Work out the finished part from the listing and answer in its coordinate system (mm). A direction names the side the tool comes from. Give positions to 0.01 mm unless a question says otherwise; leave off trailing zeros. Write each loop counter-clockwise with the first axis right and the second up, starting at its lowest first coordinate (ties: lowest second). Pieces come first, ordered by that corner, then holes. Notation, with made-up numbers: (19.25, 43.5) -> (37.25, 43.5) arc R28 cw to (37.25, 63.5) -> close; hole circle Ø8 at (76, 67.25). An arc over 180 degrees is marked (long way). Use a Markdown table: item, result. Add a question column.
Q1. For a pull along Z with two mould halves and no side action, classify faces 1 (the face through (9.63, 2.69, 22.18)), 2 (the face through (6, 6, 0)), 3 (the face through (6, 6, 35)) as pulls with the +Z half, pulls with the -Z half, needs draft (parallel to the pull), parting line crosses it, or undercut.
Q2. For faces 4 (the face through (9, 2.3, 24.4)), 5 (the face through (1.78, 9.22, 24.35)), 6 (the face through (9, 1, 23)), determine the directions among +Z, -Z, +X, -X, +Y, -Y from which every point of the face is accessible in a straight line to the end or side of a thin tool.
Q3. Section A-A, the plane x = 4.5 is taken. Give the vertices of the cut face in (y, z), plus the area to 3 significant figures.
Q4. Consider line 1 (Z direction, x = 4.5, y = 7.25); line 2 (Y direction, x = 3, z = 7); line 3 (Y direction, x = 8.75, z = 39). Determine where each line is inside the solid, lowest interval first.
Q5. Each of these flat-tipped pins is pushed along its axis until it touches: pin 1 Ø6 at (x, z) = (9, 14) entering from +Y; pin 2 Ø5 at (y, z) = (6.5, 8) entering from -X; pin 3 Ø2 at (y, z) = (2, 39.5) entering from +X; pin 4 Ø1 at (x, z) = (7.5, 29.5) entering from +Y. Where does it stop, or does it pass through?
Q6. Section C-C, the plane z = 16 is taken. Give the vertices of the cut face in (x, y), plus the area to 3 significant figures.
Q7. Section D-D, the plane z = 38 is taken. Give the vertices of the cut face in (x, y), plus the area to 3 significant figures.
Q8. Section B-B, the plane y = 3.75 is taken. Give the vertices of the cut face in (x, z), plus the area to 3 significant figures.
from build123d import *

# Parameters (mm, degrees)
DODANIE_WYCI_GNI_CIE1_DEPTH = 45
WYTNIJ_WYCI_GNI_CIE1_DEPTH  = 60
SZKIC4_W                    = 21
SZKIC4_H                    = 10
WYTNIJ_WYCI_GNI_CIE2_DEPTH  = 60


with BuildPart() as part:
    # Szkic1 → Dodanie-wyciągnięcie1 (new body)
    with BuildSketch(Plane.XY):
        with BuildLine():
            Line((0, 0), (0, 10))
            ThreePointArc((0, 10), (7.071067812, 7.071067812), (10, 0))
            Line((10, 0), (0, 0))
        make_face()
    extrude(amount=DODANIE_WYCI_GNI_CIE1_DEPTH)

    # Szkic2 → Wytnij-wyciągnięcie1 (cut)
    with BuildSketch(Plane.XY.offset(45)):
        Polygon((0, 10), (10, 0), (0, 0), align=None)
    extrude(amount=-WYTNIJ_WYCI_GNI_CIE1_DEPTH, mode=Mode.SUBTRACT)

    # Szkic4 → Wytnij-wyciągnięcie2 (cut)
    with BuildSketch(Plane(origin=(5, 5, 0), x_dir=(0, 0, 1), z_dir=(-0.707106781, -0.707106781, 0))):
        with Locations((24.5, 0.262214186)):
            Rectangle(SZKIC4_W, SZKIC4_H)
    extrude(amount=-WYTNIJ_WYCI_GNI_CIE2_DEPTH, mode=Mode.SUBTRACT)


solid = part.part
Result set:
| question | item | result |
|---|---|---|
| 1 | face 1 | needs draft |
| 1 | face 2 | pulls with the -Z half |
| 1 | face 3 | undercut |
| 2 | face 4 | -X, +Y |
| 2 | face 5 | +X, -Y |
| 2 | face 6 | +Z, -Z, -X, -Y |
| 3 | outline | (5.5, 0) -> (8.93, 0) -> (8.93, 14) -> (5.5, 14) -> close; (5.5, 35) -> (8.93, 35) -> (8.93, 45) -> (5.5, 45) -> close |
| 3 | area | 82.3 mm2 |
| 4 | line 1 | z = 0 to 14, 35 to 45 |
| 4 | line 2 | y = 7 to 9.54 |
| 4 | line 3 | y = 1.25 to 4.84 |
| 5 | pin 1 | stops at y = 8 |
| 5 | pin 2 | stops at x = 1 |
| 5 | pin 3 | stops at x = 9.95 |
| 5 | pin 4 | passes through |
| 6 | outline | (0, 10) -> (1.28, 8.72) -> (2.29, 9.73) arc R10 ccw to start; (8.35, 1.65) -> (10, 0) arc R10 ccw to (9.58, 2.88) -> close |
| 6 | area | 3.63 mm2 |
| 7 | outline | (0, 10) -> (10, 0) arc R10 ccw to start |
| 7 | area | 28.5 mm2 |
| 8 | outline | (6.25, 0) -> (9.27, 0) -> (9.27, 14) -> (6.25, 14) -> close; (6.25, 35) -> (9.27, 35) -> (9.27, 45) -> (6.25, 45) -> close |
| 8 | area | 72.5 mm2 |
